from build123d import *

# Parameters (mm, degrees)
SKETCH6_W            = 48
SKETCH6_H            = 28
SKETCH6_W_2          = 42
SKETCH6_H_2          = 21
BOSS_EXTRUDE20_DEPTH = 22
SKETCH9_W            = 48
SKETCH9_H            = 28
BOSS_EXTRUDE22_DEPTH = 2
FILLET1_R            = 2
SKETCH11_W           = 36
SKETCH11_H           = 6
BOSS_EXTRUDE23_DEPTH = 2
FILLET2_R            = 2
SKETCH12_W           = 3
SKETCH12_H           = 10
CUT_EXTRUDE2_DEPTH   = 22


with BuildPart() as part:
    # Sketch6 → Boss-Extrude20 (new body)
    with BuildSketch(Plane(origin=(0, 0, 0), x_dir=(-1, 0, 0), z_dir=(0, 1, 0))):
        with Locations((-3.5, -2.5)):
            Rectangle(SKETCH6_W, SKETCH6_H)
        with Locations((-3.5, -2.5)):
            Rectangle(SKETCH6_W_2, SKETCH6_H_2, mode=Mode.SUBTRACT)
    extrude(amount=-BOSS_EXTRUDE20_DEPTH)

    # Sketch9 → Boss-Extrude22 (add)
    with BuildSketch(Plane(origin=(0, 0, 0), x_dir=(-1, 0, 0), z_dir=(0, 1, 0))):
        with Locations((-3.5, -2.5)):
            Rectangle(SKETCH9_W, SKETCH9_H)
    extrude(amount=BOSS_EXTRUDE22_DEPTH)

    # Fillet1
    fillet1_edges = [part.edges().sort_by_distance(p)[0] for p in [
        (27.5, -10, 11.5),
        (-20.5, -10, 11.5),
        (-20.5, -10, -16.5),
        (27.5, -10, -16.5),
    ]]
    fillet(fillet1_edges, radius=FILLET1_R)

    # Sketch11 → Boss-Extrude23 (add)
    with BuildSketch(Plane(origin=(0, 2, 0), x_dir=(1, 0, 0), z_dir=(0, 1, 0))):
        with Locations((3.5, 19.5)):
            Rectangle(SKETCH11_W, SKETCH11_H)
        with Locations((3.5, -14.5)):
            Rectangle(SKETCH11_W, SKETCH11_H)
    extrude(amount=-BOSS_EXTRUDE23_DEPTH)

    # Fillet2
    fillet2_edges = [part.edges().sort_by_distance(p)[0] for p in [
        (-14.5, 1, -22.5),
        (21.5, 1, -22.5),
        (21.5, 1, 17.5),
        (-14.5, 1, 17.5),
    ]]
    fillet(fillet2_edges, radius=FILLET2_R)

    # Sketch12 → Cut-Extrude2 (cut)
    with BuildSketch(Plane.XZ.offset(22)):
        with Locations((26, -2.5)):
            Rectangle(SKETCH12_W, SKETCH12_H)
    extrude(amount=-CUT_EXTRUDE2_DEPTH, mode=Mode.SUBTRACT)


solid = part.part
Geometry: final body of the model. Coordinates: model frame, mm. A direction names the side the tool comes from. Give positions to 0.01 mm unless a question says otherwise; leave off trailing zeros. Write each loop counter-clockwise with the first axis right and the second up, starting at its lowest first coordinate (ties: lowest second). Pieces come first, ordered by that corner, then holes. Notation, with made-up numbers: (44, -9.75) -> (52, -9.75) arc R27 cw to (52, 10.25) -> close; hole circle Ø3 at (21, 36.5). An arc over 180 degrees is marked (long way). Answer in a Markdown table with one row per item.
(1) Draft query along X for faces 1 (the flat face through (-17.5, -11, -3)), 2 (the cylindrical face through (26.93, -9.83, -15.9)), 3 (the flat face through (3, 0, 14)). Return one class per face: +X half, -X half, draft (parallel to the pull), parting line (faces both ways), or undercut.
Answers below:
| item | result |
|---|---|
| face 1 | undercut |
| face 2 | +X half |
| face 3 | draft |
(2) Ray query, line 1 along Z through (x, y) = (-14, -3); line 2 along X through (y, z) = (-2.75, -8); line 3 along Y through (x, z) = (-5, -19). Return the intervals inside material, ascending. Write a range as [from, to].
Answers below:
| item | result |
|---|---|
| line 1 | [-16.5, -13], [8, 11.5] |
| line 2 | [-20.5, -17.5], [24.5, 27.5] |
| line 3 | [0, 2] |
(3) Pin query (flat end, axial travel): pin 1 (2 mm diameter, centred on y = 1.5, z = 13.5, fed in from +X); pin 2 (1.6 mm diameter, centred on y = 1, z = -17.5, fed in from -X); pin 3 (2.5 mm diameter, centred on x = 26, y = -9, fed in from +Z). Return the tip coordinate at first contact, or that it passes through.
Answers below:
| item | result |
|---|---|
| pin 1 | x = 21.5 |
| pin 2 | x = -14.5 |
| pin 3 | z = 11.5 |
(4) Section query C-C on z = -4. Return loops of the section in (x, y).
Answers below:
| item | result |
|---|---|
| outline | (-20.5, -22) -> (-17.5, -22) -> (-17.5, 0) -> (27.5, 0) -> (27.5, 2) -> (-20.5, 2) -> close |
(5) Set-up query: faces 4 (the cylindrical face through (20.93, 0.99, 16.9)), 5 (the flat face through (27.5, -10, -8)), 6 (the flat face through (24.5, -11, 5)), 7 (the flat face through (26, -11, 2.5)), 8 (the flat face through (-14.5, 1, -18)). Return all of +Z, -Z, +X, -X, +Y, -Y with unobstructed straight access to the full face (end or side cutting, diameter ignored); none if empty.
Answers below:
| item | result |
|---|---|
| face 4 | +Z, +X, +Y, -Y |
| face 5 | +Z, -Z, +X, +Y, -Y |
| face 6 | -Y |
| face 7 | +X, -Y |
| face 8 | -Z, -X, +Y, -Y |
(6) Section query B-B on x = 13.5. Return loops of the section in (y, z), then the cut area to 3 significant figures.
Answers below:
| item | result |
|---|---|
| outline | (-22, -16.5) -> (0, -16.5) -> (0, -22.5) -> (2, -22.5) -> (2, 17.5) -> (0, 17.5) -> (0, 11.5) -> (-22, 11.5) -> (-22, 8) -> (0, 8) -> (0, -13) -> (-22, -13) -> close |
| area | 234 mm^2 |
(7) Section query D-D on z = -8.5. Return loops of the section in (x, y).
Answers below:
| item | result |
|---|---|
| outline | (-20.5, -22) -> (-17.5, -22) -> (-17.5, 0) -> (24.5, 0) -> (24.5, -22) -> (27.5, -22) -> (27.5, 2) -> (-20.5, 2) -> close |
(8) Section query A-A on y = -12.75. Return loops of the section in (x, z), then the cut area to 3 significant figures.
Answers below:
| item | result |
|---|---|
| outline | (-20.5, -14.5) arc R2 ccw to (-18.5, -16.5) -> (25.5, -16.5) arc R2 ccw to (27.5, -14.5) -> (27.5, -7.5) -> (24.5, -7.5) -> (24.5, -13) -> (-17.5, -13) -> (-17.5, 8) -> (24.5, 8) -> (24.5, 2.5) -> (27.5, 2.5) -> (27.5, 9.5) arc R2 ccw to (25.5, 11.5) -> (-18.5, 11.5) arc R2 ccw to (-20.5, 9.5) -> close |
| area | 429 mm^2 |
